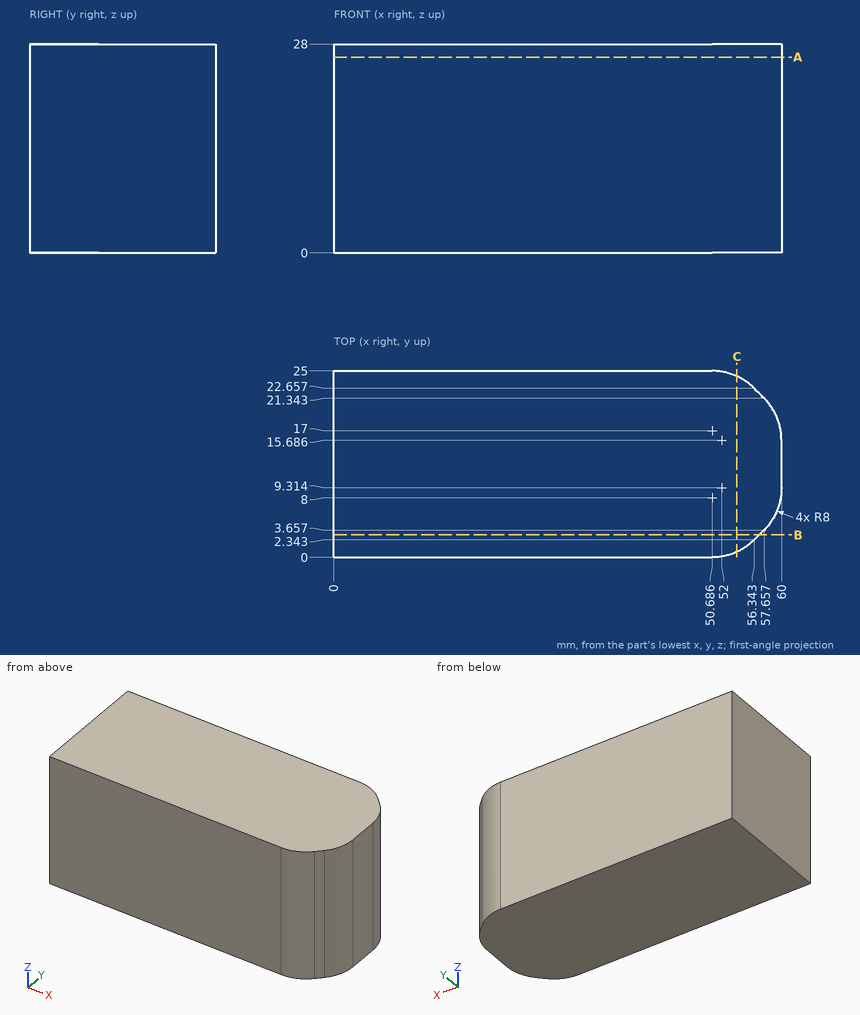
Check sheet for the drawn part. Datum: minimum x, y, z corner. Units: mm. Coordinates: 2 decimals unless noted, no trailing zeros. Write each loop counter-clockwise with the first axis right and the second up, starting at its lowest first coordinate (ties: lowest second). Pieces come first, ordered by that corner, then holes. Notation, with made-up numbers: (55.5, 6) - (78.5, 6) arc R35 cw to (78.5, 42) - close; hole circle Ø2 at (-26.5, -27.5). An arc over 180 degrees is marked (long way). Answer as a JSON object with one key per item and string values.
(1) Cross-section at C-C on x = 54. Record the cut outline in (y, z).
Report:
{"outline": "(0.72, 0) - (24.28, 0) - (24.28, 28) - (0.72, 28) - close"}
(2) Cross-section at B-B on y = 3. Record the cut outline in (x, z).
Report:
{"outline": "(0, 0) - (57, 0) - (57, 28) - (0, 28) - close"}
(3) Gauge pin test, flat end, axial feed: pin 1 Ø4 at (y, z) = (4, 8) entering from -X. Record the tip position at first contact, or that the pin passes through.
Report:
{"pin 1": "x = 0"}
(4) Thickness scan on line 1 along Y through (x, z) = (55, 18.5); line 2 along X through (y, z) = (2.25, 14.25); line 3 along X through (y, z) = (18, 10.5). Record the ranges inside material, lowest first.
Report:
{"line 1": "1.26 to 23.74", "line 2": "0 to 56.25", "line 3": "0 to 59.66"}
(5) Cross-section at A-A on z = 26.25. Record the cut outline in (x, y).
Report:
{"outline": "(0, 0) - (50.69, 0) arc R8 ccw to (56.34, 2.34) - (57.66, 3.66) arc R8 ccw to (60, 9.31) - (60, 15.69) arc R8 ccw to (57.66, 21.34) - (56.34, 22.66) arc R8 ccw to (50.69, 25) - (0, 25) - close"}
